The listing builds one solid part. Answer for the finished solid, in the listing's coordinates (mm). Face numbers are marked on the shaded views. A direction names the side the tool comes from. Coordinates: 2 decimals unless noted, no trailing zeros. Order: outer loops, then holes, each group sorted by start corner. A loop starts at its lowest first (then second) coordinate and runs counter-clockwise, first axis right, second up. Notation, with made-up numbers: (42, 34.25) - (87, 34.25) arc R20 cw to (87, 64.25) - close; hole circle Ø11 at (52, 73). An arc over 180 degrees is marked (long way). Use one line per item in the form item = value. Start each with the question number.
Item 1: This flat-tipped pin is pushed along its axis until it touches: pin 1 Ø2 at (x, z) = (21, -8) entering from +Y. Where does it stop, or does it pass through?
Item 2: Section B-B, the plane z = -8 is taken. Write down the section's boundary in (x, y), and give its area (3 significant figures).
Item 3: Section A-A, the plane x = 2.5 is taken. Write down the section's boundary in (y, z), and give its area (4 significant figures).
Item 4: A tool of negligible diameter and unlimited length cuts with its end or side. For the marked faces 1 and 2, from which of +Z, -Z, +X, -X, +Y, -Y can it reach the whole face along a straight path? Write none if from no direction.
Item 5: Section D-D, the plane z = -14.25 is taken. Write down the section's boundary in (x, y), and give its area (3 significant figures).
Item 6: The mould has two halves that part along X. Classify the marked faces 3, 4, 5 and 6: released by +X, released by -X, zero draft, split by the parting line, or undercut.
Item 7: Section C-C, the plane x = 21 is taken. Write down the section's boundary in (y, z), and give its area (3 significant figures).
Item 8: Consider line 1 along Z through (x, y) = (2.5, 1.95); line 2 along Y through (x, z) = (3.75, -7.5); line 3 along Y through (x, z) = (7.75, -12.5). Determine where each line is inside the solid, lowest interval first. Write a range as [from, to].
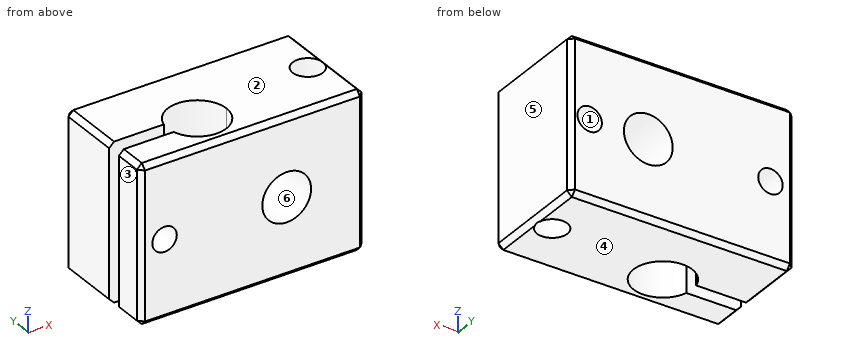
from build123d import *

# Parameters (mm, degrees)
SKETCH1_W                  = 23
SKETCH1_H                  = 16
BOSS_EXTRUDE1_DEPTH        = 11.5
SKETCH10_R                 = 1.55
CUT_EXTRUDE2_DEPTH         = 31.286135442
M3X0_5_TAPPED_HOLE1_REACH  = 32.286
M3X0_5_TAPPED_HOLE1_BORE_R = 1.25
M6_TAPPED_HOLE1_D          = 5
CUT_EXTRUDE1_DEPTH         = 16


with BuildPart() as part:
    # Sketch1 → Boss-Extrude1 (new body)
    with BuildSketch(Plane(origin=(0, 0, 0), x_dir=(1, 0, 0), z_dir=(0, 1, 0))):
        with Locations((11.5, 8)):
            Rectangle(SKETCH1_W, SKETCH1_H)
    extrude(amount=BOSS_EXTRUDE1_DEPTH)

    # Sketch10 → Cut-Extrude2 (cut, through all)
    with BuildSketch(Plane.XY):
        with Locations((21, 5.75)):
            Circle(SKETCH10_R)
    extrude(amount=-CUT_EXTRUDE2_DEPTH, mode=Mode.SUBTRACT)

    # M3x0.5 Tapped Hole1 bore → M3x0.5 Tapped Hole1 (cut, up to next)
    with BuildSketch(Plane(origin=(0, 11.5, 0), x_dir=(1, 0, 0), z_dir=(0, 1, 0)), mode=Mode.PRIVATE) as m3x0_5_tapped_hole1_sk1:
        with Locations((2.5, 8)):
            Circle(M3X0_5_TAPPED_HOLE1_BORE_R)
    m3x0_5_tapped_hole1_tool1 = extrude(m3x0_5_tapped_hole1_sk1.sketch, amount=-M3X0_5_TAPPED_HOLE1_REACH, mode=Mode.PRIVATE) & part.part
    # M3x0.5 Tapped Hole1 bore → M3x0.5 Tapped Hole1 (cut, up to next)
    with BuildSketch(Plane(origin=(0, 11.5, 0), x_dir=(1, 0, 0), z_dir=(0, 1, 0)), mode=Mode.PRIVATE) as m3x0_5_tapped_hole1_sk2:
        with Locations((21, 8)):
            Circle(M3X0_5_TAPPED_HOLE1_BORE_R)
    m3x0_5_tapped_hole1_tool2 = extrude(m3x0_5_tapped_hole1_sk2.sketch, amount=-M3X0_5_TAPPED_HOLE1_REACH, mode=Mode.PRIVATE) & part.part
    add(m3x0_5_tapped_hole1_tool1.solids().sort_by_distance((2.5, 11.5, -8))[0], mode=Mode.SUBTRACT)
    add(m3x0_5_tapped_hole1_tool2.solids().sort_by_distance((21, 11.5, -8))[0], mode=Mode.SUBTRACT)

    # M6 Tapped Hole1 (through all)
    with Locations(Plane(origin=(0, 11.5, 0), x_dir=(1, 0, 0), z_dir=(0, 1, 0))):
        with Locations((15, 8)):
            Hole(M6_TAPPED_HOLE1_D / 2)

    # Sketch2 → Cut-Extrude1 (cut)
    with BuildSketch(Plane.XY):
        with BuildLine():
            Line((5.59526249, 4.75), (0, 4.75))
            Line((0, 4.75), (0, 3.25))
            Line((0, 3.25), (5.59526249, 3.25))
            ThreePointArc((5.59526249, 3.25), (5.5, 4), (5.59526249, 4.75))
        make_face()
        with BuildLine():
            ThreePointArc((11.5, 4), (8.878012877, 6.976089089), (5.59526249, 4.75))
            Line((5.59526249, 4.75), (5.59526249, 3.25))
            ThreePointArc((5.59526249, 3.25), (8.878012877, 1.023910911), (11.5, 4))
        make_face()
        with BuildLine():
            Line((5.59526249, 3.25), (5.59526249, 4.75))
            ThreePointArc((5.59526249, 4.75), (5.5, 4), (5.59526249, 3.25))
        make_face()
    extrude(amount=-CUT_EXTRUDE1_DEPTH, mode=Mode.SUBTRACT)

    # Chamfer1
    # the kernel refuses this chamfer: 0.5 mm, written as the material it takes off along each edge
    with BuildSketch(Plane(origin=(22.666666667, 11.166666667, -0.333333333), x_dir=(0.7071067811865475, 0, -0.7071067811865475), z_dir=(0.5773502691896258, 0.5773502691896258, 0.5773502691896258)), Plane(origin=(0.333333333, 0.333333333, -0.333333333), x_dir=(-0.7071067811865475, 0, -0.7071067811865475), z_dir=(-0.5773502691896257, -0.5773502691896257, 0.5773502691896257)), Plane(origin=(0.333333333, 11.166666667, -0.333333333), x_dir=(0, 0.7071067811865476, -0.7071067811865475), z_dir=(-0.5773502691896258, 0.5773502691896257, 0.5773502691896258)), Plane(origin=(22.666666667, 0.333333333, -15.666666667), x_dir=(0, 0.7071067811865475, -0.7071067811865475), z_dir=(0.5773502691896258, -0.5773502691896258, -0.5773502691896258)), Plane(origin=(22.666666667, 0.333333333, -0.333333333), x_dir=(0, -0.7071067811865475, -0.7071067811865475), z_dir=(0.5773502691896258, -0.5773502691896258, 0.5773502691896258))) as chamfer1_piece_1:
        Polygon((-0.353553391, -0.204124145), (0.353553391, -0.204124145), (0, 0.40824829), align=None)
    extrude(amount=0.635085296, mode=Mode.SUBTRACT)
    with BuildSketch(Plane(origin=(22.666666667, 11.166666667, -15.666666667), x_dir=(0.7071067811865475, 0, 0.7071067811865475), z_dir=(0.5773502691896258, 0.5773502691896258, -0.5773502691896258)), Plane(origin=(0.333333333, 11.166666667, -15.666666667), x_dir=(0, 0.7071067811865475, 0.7071067811865475), z_dir=(-0.5773502691896258, 0.5773502691896257, -0.5773502691896258)), Plane(origin=(0.333333333, 0.333333333, -15.666666667), x_dir=(0.7071067811865475, -0.7071067811865475, 0), z_dir=(-0.5773502691896257, -0.5773502691896257, -0.5773502691896258))) as chamfer1_piece_2:
        Polygon((-0.353553391, 0.204124145), (0.353553391, 0.204124145), (0, -0.40824829), align=None)
    extrude(amount=0.635085296, mode=Mode.SUBTRACT)
    with BuildSketch(Plane(origin=(23, 11.5, 1.285841494), x_dir=(0.0274958766105891, -0.9996219169112968, 0), z_dir=(0, 0, -1)), Plane(origin=(23, 0, 1.285841494), x_dir=(-0.9996219169112968, -0.027495876610586292, 0), z_dir=(0, 0, -1)), Plane(origin=(0, 0, -17.285841494), x_dir=(0.9996219169112968, -0.027495876610586372, 0), z_dir=(0, 0, 1))) as chamfer1_piece_3:
        with BuildLine():
            Line((0.514336598, 0), (-0.028273577, 0.513558897))
            Line((-0.028273577, 0.513558897), (-0.038269797, 0.513283938))
            ThreePointArc((-0.038269797, 0.513283938), (-0.017064614, 0.256698915), (-0.009996219, -0.000274959))
            Line((-0.009996219, -0.000274959), (0.000274959, -0.009996219))
            ThreePointArc((0.000274959, -0.009996219), (0.257248832, -0.002927825), (0.514611556, -0.009996219))
            Line((0.514611556, -0.009996219), (0.514336598, 0))
        make_face()
    extrude(amount=18.571682988, mode=Mode.SUBTRACT)
    with BuildSketch(Plane(origin=(24.285841494, 11.5, -16), x_dir=(0, 0.027495876610585647, 0.9996219169112968), z_dir=(-1, 0, 0)), Plane(origin=(-1.285841494, 0, 0), x_dir=(0, 0.9996219169112968, 0.027495876610586372), z_dir=(1, 0, 0))) as chamfer1_piece_4:
        with BuildLine():
            Line((0.514336598, 0), (-0.028273577, -0.513558897))
            Line((-0.028273577, -0.513558897), (-0.038269797, -0.513283938))
            ThreePointArc((-0.038269797, -0.513283938), (-0.017064614, -0.256698915), (-0.009996219, 0.000274959))
            Line((-0.009996219, 0.000274959), (0.000274959, 0.009996219))
            ThreePointArc((0.000274959, 0.009996219), (0.257248832, 0.002927825), (0.514611556, 0.009996219))
            Line((0.514611556, 0.009996219), (0.514336598, 0))
        make_face()
    extrude(amount=25.571682988, mode=Mode.SUBTRACT)
    with BuildSketch(Plane(origin=(0, -1.285841494, -16), x_dir=(-0.02749587661058639, 0, 0.9996219169112968), z_dir=(0, 1, 0)), Plane(origin=(0, -1.285841494, 0), x_dir=(0.9996219169112968, 0, 0.027495876610586372), z_dir=(0, 1, 0))) as chamfer1_piece_5:
        with BuildLine():
            Line((0.514336598, 0), (-0.028273577, 0.513558897))
            Line((-0.028273577, 0.513558897), (-0.038269797, 0.513283938))
            ThreePointArc((-0.038269797, 0.513283938), (-0.017064614, 0.256698915), (-0.009996219, -0.000274959))
            Line((-0.009996219, -0.000274959), (0.000274959, -0.009996219))
            ThreePointArc((0.000274959, -0.009996219), (0.257248832, -0.002927825), (0.514611556, -0.009996219))
            Line((0.514611556, -0.009996219), (0.514336598, 0))
        make_face()
    extrude(amount=5.821682988, mode=Mode.SUBTRACT)
    with BuildSketch(Plane(origin=(0, 11.5, -17.285841494), x_dir=(0.9996219169112968, 0.02749587661058563, 0), z_dir=(0, 0, 1))) as chamfer1_piece_6:
        with BuildLine():
            Line((0.514336598, 0), (-0.028273577, -0.513558897))
            Line((-0.028273577, -0.513558897), (-0.038269797, -0.513283938))
            ThreePointArc((-0.038269797, -0.513283938), (-0.017064614, -0.256698915), (-0.009996219, 0.000274959))
            Line((-0.009996219, 0.000274959), (0.000274959, 0.009996219))
            ThreePointArc((0.000274959, 0.009996219), (0.257248832, 0.002927825), (0.514611556, 0.009996219))
            Line((0.514611556, 0.009996219), (0.514336598, 0))
        make_face()
    extrude(amount=18.571682988, mode=Mode.SUBTRACT)
    with BuildSketch(Plane(origin=(24.285841494, 0, -16), x_dir=(0, -0.02749587661058639, 0.9996219169112968), z_dir=(-1, 0, 0)), Plane(origin=(-1.285841494, 11.5, 0), x_dir=(0, -0.9996219169112968, 0.02749587661058639), z_dir=(1, 0, 0))) as chamfer1_piece_7:
        with BuildLine():
            Line((0.514336598, 0), (-0.028273577, 0.513558897))
            Line((-0.028273577, 0.513558897), (-0.038269797, 0.513283938))
            ThreePointArc((-0.038269797, 0.513283938), (-0.017064614, 0.256698915), (-0.009996219, -0.000274959))
            Line((-0.009996219, -0.000274959), (0.000274959, -0.009996219))
            ThreePointArc((0.000274959, -0.009996219), (0.257248832, -0.002927825), (0.514611556, -0.009996219))
            Line((0.514611556, -0.009996219), (0.514336598, 0))
        make_face()
    extrude(amount=25.571682988, mode=Mode.SUBTRACT)
    with BuildSketch(Plane(origin=(0, 3.464158506, -16), x_dir=(-0.02749587661058639, 0, 0.9996219169112968), z_dir=(0, 1, 0)), Plane(origin=(0, 3.464158506, 0), x_dir=(0.9996219169112968, 0, 0.027495876610586372), z_dir=(0, 1, 0))) as chamfer1_piece_8:
        with BuildLine():
            Line((0.514336598, 0), (-0.028273577, 0.513558897))
            Line((-0.028273577, 0.513558897), (-0.038269797, 0.513283938))
            ThreePointArc((-0.038269797, 0.513283938), (-0.017064614, 0.256698915), (-0.009996219, -0.000274959))
            Line((-0.009996219, -0.000274959), (0.000274959, -0.009996219))
            ThreePointArc((0.000274959, -0.009996219), (0.257248832, -0.002927825), (0.514611556, -0.009996219))
            Line((0.514611556, -0.009996219), (0.514336598, 0))
        make_face()
    extrude(amount=9.321682988, mode=Mode.SUBTRACT)
    with BuildSketch(Plane(origin=(23, -1.285841494, -16), x_dir=(0.0274958766105891, 0, 0.9996219169112968), z_dir=(0, 1, 0)), Plane(origin=(23, -1.285841494, 0), x_dir=(-0.9996219169112968, 0, 0.027495876610586292), z_dir=(0, 1, 0))) as chamfer1_piece_9:
        with BuildLine():
            Line((0.514336598, 0), (-0.028273577, -0.513558897))
            Line((-0.028273577, -0.513558897), (-0.038269797, -0.513283938))
            ThreePointArc((-0.038269797, -0.513283938), (-0.017064614, -0.256698915), (-0.009996219, 0.000274959))
            Line((-0.009996219, 0.000274959), (0.000274959, 0.009996219))
            ThreePointArc((0.000274959, 0.009996219), (0.257248832, 0.002927825), (0.514611556, 0.009996219))
            Line((0.514611556, 0.009996219), (0.514336598, 0))
        make_face()
    extrude(amount=14.071682988, mode=Mode.SUBTRACT)


solid = part.part
Response:
q1.pin_1 = 4.57
q2.outline = (0, 0.5) - (0.5, 0) - (1.25, 0) - (1.25, 3.25) - (0, 3.25) - close; (0, 4.75) - (1.25, 4.75) - (1.25, 11.5) - (0.5, 11.5) - (0, 11) - close; (3.75, 0) - (12.5, 0) - (12.5, 11.5) - (3.75, 11.5) - (3.75, 4.75) - (5.6, 4.75) arc R3 cw (long way) to (5.6, 3.25) - (3.75, 3.25) - close; (17.5, 0) - (22.5, 0) - (23, 0.5) - (23, 11) - (22.5, 11.5) - (22.25, 11.5) - (22.25, 6.67) arc R1.55 cw (long way) to (19.75, 6.67) - (19.75, 11.5) - (17.5, 11.5) - close
q2.area = 126 mm2
q3.outline = (0, -15.5) - (0.5, -16) - (3.25, -16) - (3.25, -9.25) - (0, -9.25) - close; (0, -6.75) - (3.25, -6.75) - (3.25, 0) - (0.5, 0) - (0, -0.5) - close; (4.75, -16) - (11, -16) - (11.5, -15.5) - (11.5, -9.25) - (4.75, -9.25) - close; (4.75, -6.75) - (11.5, -6.75) - (11.5, -0.5) - (11, 0) - (4.75, 0) - close
q3.area = 134.5 mm2
q4.face_1 = +Y
q4.face_2 = +Z, +X, -X, +Y, -Y
q5.outline = (0, 0.5) - (0.5, 0) - (22.5, 0) - (23, 0.5) - (23, 11) - (22.5, 11.5) - (0.5, 11.5) - (0, 11) - (0, 4.75) - (5.6, 4.75) arc R3 cw (long way) to (5.6, 3.25) - (0, 3.25) - close; hole circle Ø3.1 at (21, 5.75)
q5.area = 220 mm2
q6.face_3 = released by -X
q6.face_4 = zero draft
q6.face_5 = released by +X
q6.face_6 = undercut
q7.outline = (0, -15.5) - (0.5, -16) - (4.2, -16) - (4.2, 0) - (0.5, 0) - (0, -0.5) - close; (7.3, -16) - (11, -16) - (11.5, -15.5) - (11.5, -9.25) - (7.3, -9.25) - close; (7.3, -6.75) - (11.5, -6.75) - (11.5, -0.5) - (11, 0) - (7.3, 0) - close
q7.area = 123 mm2
q8.line_1 = [-16, -9.25], [-6.75, 0]
q8.line_2 = [0, 3.25], [4.75, 11.5]
q8.line_3 = [0, 1.1], [6.9, 11.5]
